from build123d import *

# Parameters (mm, degrees)
F0_R     = 10
F1_DEPTH = 25
F2_R     = 10
F3_DEPTH = 50
F4_SIZE  = 2


with BuildPart() as f1:
    # F0 (on Front) → F1 (new body)
    with BuildSketch(Plane.XZ):
        with BuildLine():
            ThreePointArc((2.100041, 24.91164), (-24.999999, 0.008383), (2.083333, -24.913043))
            ThreePointArc((2.083333, -24.913043), (18.399502, -16.92508), (25, 0))
            ThreePointArc((25, 0), (18.405176, 16.918909), (2.100041, 24.91164))
        make_face()
        Circle(F0_R, mode=Mode.SUBTRACT)
        with BuildLine():
            ThreePointArc((25, 0), (18.399502, -16.92508), (2.083333, -24.913043))
            Line((2.083333, -24.913043), (91.458333, -17.43913))
            ThreePointArc((91.458333, -17.43913), (72.514802, -0.71961), (90.020401, 17.499988))
            Line((90.020401, 17.499988), (2.100041, 24.91164))
            ThreePointArc((2.100041, 24.91164), (18.405176, 16.918909), (25, 0))
        make_face()
        with BuildLine():
            ThreePointArc((90.020401, 17.499988), (72.514802, -0.71961), (91.458333, -17.43913))
            ThreePointArc((91.458333, -17.43913), (102.879651, -11.847556), (107.5, 0))
            ThreePointArc((107.5, 0), (102.381579, 12.367154), (90.020401, 17.499988))
        make_face()
        with Locations((90, 0)):
            Circle(F0_R, mode=Mode.SUBTRACT)
    extrude(amount=F1_DEPTH)

    # F2 (on face) → F3 (join)
    with BuildSketch(Plane.XZ):
        with BuildLine():
            ThreePointArc((25, 0), (18.405176, 16.918909), (2.100041, 24.91164))
            ThreePointArc((2.100041, 24.91164), (-24.999999, 0.008383), (2.083333, -24.913043))
            ThreePointArc((2.083333, -24.913043), (18.399502, -16.92508), (25, 0))
        make_face()
        Circle(F2_R, mode=Mode.SUBTRACT)
    extrude(amount=F3_DEPTH)

    # F4
    f4_edges = [f1.edges().sort_by_distance(p)[0] for p in [
        (-2.083333, -50, 24.913043),
        (-10, -50, 0),
        (80, -25, 0),
    ]]
    chamfer(f4_edges, length=F4_SIZE)


solid = f1.part
The model under review builds one solid part; all positions refer to its coordinate system, in mm. Coordinates: 2 decimals unless noted, no trailing zeros. Loops run counter-clockwise (first coordinate to the right, second up) from the corner with the lowest first, then second, coordinate; pieces in that order, holes last. Notation, with made-up numbers: M 72,25.5 L 129,25.5 A27 cw 129,49.5 Z; hole C 49,81.25 d2. An arc over 180 degrees is marked long. Put each result on its own line as item: value. Start each with the question number.
Q1. The part is to be moulded in two halves that separate along X. For faces 1 (the flat face through (40, 0, 0)), 2 (the flat face through (46.15, -12.32, -21.23)), 3 (the cylindrical face through (-2.17, -23.66, -9.76)), say which applies: +X half, -X half, draft (parallel to the pull), parting line (faces both ways), or undercut.
Q2. Clearance check with flat-ended pins moving along their axes: pin 1 (4 mm diameter, centred on y = -39.5, z = 11, fed in from -X); pin 2 (15 mm diameter, centred on x = 43.5, z = 7, fed in from -Y); pin 3 (1.5 mm diameter, centred on x = -2.5, z = 8.5, fed in from -Y); pin 4 (1.5 mm diameter, centred on x = -11.5, y = -37, fed in from +Z). State where each tip first meets the part, or that it passes through.
Q3. Add section C-C (x = 65.5). Write out the cut boundary in (y, z), and give its area (3 significant figures).
Q4. Add section B-B (z = -1.5). Count the separate pieces of the cut face and the enclosed holes in it, and give its area (3 significant figures).
Q5. Add section A-A (y = -42.5). Write out the cut boundary in (x, z).
Q6. Wall thickness on line 1 (Z direction, x = 0, y = -24); line 2 (X direction, y = -12.5, z = -8); line 3 (Y direction, x = 24.5, z = 18): over which ranges is each line inside the solid? List them lowest first.
Q7. Add section D-D (x = 35.5). Write out the cut boundary in (y, z).
Answers:
1. face 1: draft
1. face 2: +X half
1. face 3: undercut
2. pin 1: stops at x = -23.32
2. pin 2: stops at y = -25
2. pin 3: passes through
2. pin 4: stops at z = 22.57
3. outline: M -25,-19.61 L 0,-19.61 L 0,19.57 L -25,19.57 Z
3. area: 979 mm^2
4. separate pieces: 3
4. enclosed holes: 0
4. area: 3,060 mm^2
5. outline: C 0,0 d50; hole C 0,0 d20
6. line 1: z = -25 to -10, 10 to 25
6. line 2: x = -23.69 to -6, 6 to 84, 96 to 105.56
6. line 3: y = -25 to 0
7. outline: M -25,-22.12 L 0,-22.12 L 0,22.1 L -25,22.1 Z
